Read the model definition and answer for the solid it produces. Units are mm, in the model's axes. A direction names the side the tool comes from. Give positions to 0.01 mm unless a question says otherwise; leave off trailing zeros. Write each loop counter-clockwise with the first axis right and the second up, starting at its lowest first coordinate (ties: lowest second). Pieces come first, ordered by that corner, then holes. Notation, with made-up numbers: M -6.5,26 L 35.5,26 A24 cw 35.5,40 Z; hole C 64,3 d5. An arc over 180 degrees is marked long. Put each result on its own line as item: value.
from build123d import *

# Parameters (mm, degrees)
SKETCH1_W           = 386.08
SKETCH1_H           = 88.9
BOSS_EXTRUDE1_DEPTH = 7.112


with BuildPart() as part:
    # Sketch1 → Boss-Extrude1 (new body)
    with BuildSketch(Plane(origin=(0, 0, 0), x_dir=(1, 0, 0), z_dir=(0, 1, 0))):
        with Locations((193.04, 44.45)):
            Rectangle(SKETCH1_W, SKETCH1_H)
        with BuildLine():
            Line((73.66, 63.5), (73.66, 25.4))
            ThreePointArc((73.66, 25.4), (77.379743879, 16.419743879), (86.36, 12.7))
            Line((86.36, 12.7), (111.76, 12.7))
            ThreePointArc((111.76, 12.7), (120.740256121, 16.419743879), (124.46, 25.4))
            Line((124.46, 25.4), (124.46, 63.5))
            ThreePointArc((124.46, 63.5), (120.740256121, 72.480256121), (111.76, 76.2))
            Line((111.76, 76.2), (86.36, 76.2))
            ThreePointArc((86.36, 76.2), (77.379743879, 72.480256121), (73.66, 63.5))
        make_face(mode=Mode.SUBTRACT)
        with BuildLine():
            Line((25.4, 76.2), (50.8, 76.2))
            ThreePointArc((50.8, 76.2), (59.780256121, 72.480256121), (63.5, 63.5))
            Line((63.5, 63.5), (63.5, 25.4))
            ThreePointArc((63.5, 25.4), (59.780256121, 16.419743879), (50.8, 12.7))
            Line((50.8, 12.7), (25.4, 12.7))
            ThreePointArc((25.4, 12.7), (16.419743879, 16.419743879), (12.7, 25.4))
            Line((12.7, 25.4), (12.7, 63.5))
            ThreePointArc((12.7, 63.5), (16.419743879, 72.480256121), (25.4, 76.2))
        make_face(mode=Mode.SUBTRACT)
        with BuildLine():
            Line((134.62, 63.5), (134.62, 25.4))
            ThreePointArc((134.62, 25.4), (138.339743879, 16.419743879), (147.32, 12.7))
            Line((147.32, 12.7), (172.72, 12.7))
            ThreePointArc((172.72, 12.7), (181.700256121, 16.419743879), (185.42, 25.4))
            Line((185.42, 25.4), (185.42, 63.5))
            ThreePointArc((185.42, 63.5), (181.700256121, 72.480256121), (172.72, 76.2))
            Line((172.72, 76.2), (147.32, 76.2))
            ThreePointArc((147.32, 76.2), (138.339743879, 72.480256121), (134.62, 63.5))
        make_face(mode=Mode.SUBTRACT)
        with BuildLine():
            Line((195.58, 63.5), (195.58, 25.4))
            ThreePointArc((195.58, 25.4), (199.299743879, 16.419743879), (208.28, 12.7))
            Line((208.28, 12.7), (233.68, 12.7))
            ThreePointArc((233.68, 12.7), (242.660256121, 16.419743879), (246.38, 25.4))
            Line((246.38, 25.4), (246.38, 63.5))
            ThreePointArc((246.38, 63.5), (242.660256121, 72.480256121), (233.68, 76.2))
            Line((233.68, 76.2), (208.28, 76.2))
            ThreePointArc((208.28, 76.2), (199.299743879, 72.480256121), (195.58, 63.5))
        make_face(mode=Mode.SUBTRACT)
        with BuildLine():
            Line((256.54, 63.5), (256.54, 25.4))
            ThreePointArc((256.54, 25.4), (260.259743879, 16.419743879), (269.24, 12.7))
            Line((269.24, 12.7), (294.64, 12.7))
            ThreePointArc((294.64, 12.7), (303.620256121, 16.419743879), (307.34, 25.4))
            Line((307.34, 25.4), (307.34, 63.5))
            ThreePointArc((307.34, 63.5), (303.620256121, 72.480256121), (294.64, 76.2))
            Line((294.64, 76.2), (269.24, 76.2))
            ThreePointArc((269.24, 76.2), (260.259743879, 72.480256121), (256.54, 63.5))
        make_face(mode=Mode.SUBTRACT)
        with BuildLine():
            Line((317.5, 63.5), (317.5, 25.4))
            ThreePointArc((317.5, 25.4), (321.219743879, 16.419743879), (330.2, 12.7))
            Line((330.2, 12.7), (355.6, 12.7))
            ThreePointArc((355.6, 12.7), (364.580256121, 16.419743879), (368.3, 25.4))
            Line((368.3, 25.4), (368.3, 63.5))
            ThreePointArc((368.3, 63.5), (364.580256121, 72.480256121), (355.6, 76.2))
            Line((355.6, 76.2), (330.2, 76.2))
            ThreePointArc((330.2, 76.2), (321.219743879, 72.480256121), (317.5, 63.5))
        make_face(mode=Mode.SUBTRACT)
    extrude(amount=BOSS_EXTRUDE1_DEPTH)


solid = part.part
(1) For a pull along X with two mould halves and no side action, classify faces 1 (the face through (282, 4, -12.7)), 2 (the face through (282, 4, -76.2)), 3 (the face through (190, 7.112, -45)) as +X half, -X half, draft (parallel to the pull), parting line (faces both ways), or undercut.
Result:
face 1: undercut
face 2: undercut
face 3: draft
(2) Which of the six approach directions +Z, -Z, +X, -X, +Y, -Y give full straight-line access (tool end or side, diameter ignored) to faces 4 (the face through (199.2, 3.51, -16.52)), 5 (the face through (190, 4, -88.9))?
Result:
face 4: +Y, -Y
face 5: -Z, +X, -X, +Y, -Y
(3) Section A-A on z = -42.5 is taken. Determine the outline of the cut face in (x, y).
Result:
outline: M 0,0 L 12.7,0 L 12.7,7.11 L 0,7.11 Z; M 63.5,0 L 73.66,0 L 73.66,7.11 L 63.5,7.11 Z; M 124.46,0 L 134.62,0 L 134.62,7.11 L 124.46,7.11 Z; M 185.42,0 L 195.58,0 L 195.58,7.11 L 185.42,7.11 Z; M 246.38,0 L 256.54,0 L 256.54,7.11 L 246.38,7.11 Z; M 307.34,0 L 317.5,0 L 317.5,7.11 L 307.34,7.11 Z; M 368.3,0 L 386.08,0 L 386.08,7.11 L 368.3,7.11 Z
(4) Section C-C on y = 4.75 is taken. Give the number of separate pieces and of enclosed holes in the cut face, and give its area (3 significant figures).
Result:
separate pieces: 1
enclosed holes: 6
area: 15,800 mm²
(5) Section D-D on x = 240 is taken. Determine the outline of the cut face in (y, z), and give its area (3 significant figures).
Result:
outline: M 0,-88.9 L 7.11,-88.9 L 7.11,-74.52 L 0,-74.52 Z; M 0,-14.38 L 7.11,-14.38 L 7.11,0 L 0,0 Z
area: 205 mm²
(6) Section B-B on x = 42.5 is taken. Determine the outline of the cut face in (y, z).
Result:
outline: M 0,-88.9 L 7.11,-88.9 L 7.11,-76.2 L 0,-76.2 Z; M 0,-12.7 L 7.11,-12.7 L 7.11,0 L 0,0 Z
(7) Given pin 1 Ø2 at (y, z) = (4, -47) entering from -X, flat-ended and moving along its own axis, determine where the tip first touches the part or whether it passes through.
Result:
pin 1: stops at x = 0
(8) Straight lines are drawn through the part: line 1 along Z through (x, y) = (215, 3.75); line 2 along Z through (x, y) = (265.5, 1.5). For each, find the intervals that lie inside material, in ascending order. Write a range as from..to.
Result:
line 1: z = -88.9..-76.2, -12.7..0
line 2: z = -88.9..-75.64, -13.26..0
